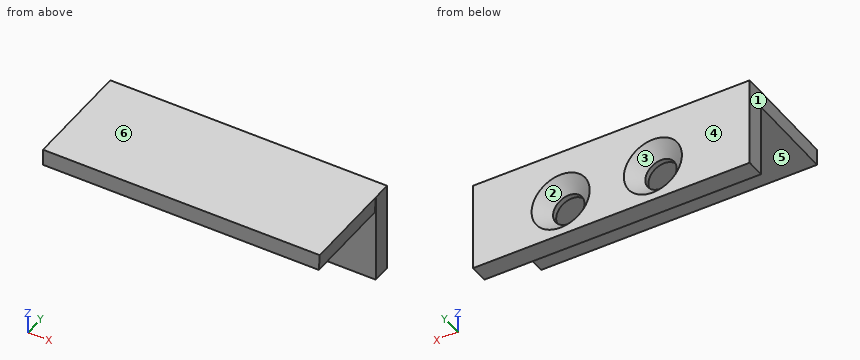
from build123d import *

# Parameters (mm, degrees)
SKIZZE1_W                                            = 30
SKIZZE1_H                                            = 9.8
AUFSATZ_LINEAR_AUSTRAGEN1_DEPTH                      = 2
FORMSENKUNG_F_R_M3_LINSENSENKSCHRAUBE_MI_D           = 3.4
FORMSENKUNG_F_R_M3_LINSENSENKSCHRAUBE_MI_DEPTH       = 8.5
FORMSENKUNG_F_R_M3_LINSENSENKSCHRAUBE_MI_CSINK_D     = 6.3
FORMSENKUNG_F_R_M3_LINSENSENKSCHRAUBE_MI_CSINK_ANGLE = 90
FORMSENKUNG_F_R_M3_LINSENSENKSCHRAUBE_MI_TIP         = 1.021463052
AUFSATZ_LINEAR_AUSTRAGEN2_DEPTH                      = 10


with BuildPart() as part:
    # Skizze1 → Aufsatz-Linear austragen1 (new body)
    with BuildSketch(Plane(origin=(0, 0, 0), x_dir=(1, 0, 0), z_dir=(0, 1, 0))):
        with Locations((5, 8.1)):
            Rectangle(SKIZZE1_W, SKIZZE1_H)
    extrude(amount=AUFSATZ_LINEAR_AUSTRAGEN1_DEPTH)

    # Formsenkung für M3 Linsensenkschraube mit Schlitz1
    with Locations(Plane(origin=(0, 2, 0), x_dir=(1, 0, 0), z_dir=(0, 1, 0))):
        with Locations((0.5, 9), (10.5, 9)):
            CounterSinkHole(FORMSENKUNG_F_R_M3_LINSENSENKSCHRAUBE_MI_D / 2, FORMSENKUNG_F_R_M3_LINSENSENKSCHRAUBE_MI_CSINK_D / 2, depth=FORMSENKUNG_F_R_M3_LINSENSENKSCHRAUBE_MI_DEPTH, counter_sink_angle=FORMSENKUNG_F_R_M3_LINSENSENKSCHRAUBE_MI_CSINK_ANGLE)
            with Locations((0, 0, -(FORMSENKUNG_F_R_M3_LINSENSENKSCHRAUBE_MI_DEPTH + FORMSENKUNG_F_R_M3_LINSENSENKSCHRAUBE_MI_TIP / 2))):  # 118° drill point
                Cone(0, FORMSENKUNG_F_R_M3_LINSENSENKSCHRAUBE_MI_D / 2, FORMSENKUNG_F_R_M3_LINSENSENKSCHRAUBE_MI_TIP, mode=Mode.SUBTRACT)

    # Skizze13 → Aufsatz-Linear austragen2 (add)
    with BuildSketch(Plane.XZ):
        Polygon((-10, -3.2), (-10, -4.99756301), (19.906366545, -4.99756301), (20, -3.2), align=None)
    extrude(amount=AUFSATZ_LINEAR_AUSTRAGEN2_DEPTH)


solid = part.part
For this review, take the finished solid that the model builds, in its own axes (mm). Face numbers are marked on the shaded views. A direction names the side the tool comes from. Give positions to 0.01 mm unless a question says otherwise; leave off trailing zeros. Loops run counter-clockwise (first coordinate to the right, second up) from the corner with the lowest first, then second, coordinate; pieces in that order, holes last. Notation, with made-up numbers: M 69.5,79.5 L 127.5,79.5 A20 cw 127.5,109.5 Z; hole C 76.5,55.25 d7. An arc over 180 degrees is marked long. Put each result on its own line as item: value. Start each with the question number.
(1) Wall thickness on L1, parallel to X at y = 0.25, z = -9; L2, parallel to Z at x = 10.5, y = 0.3; L3, parallel to Y at x = 13.5, z = -10.5: over which ranges is each line inside the solid? List them lowest first.
(2) The part is to be moulded in two halves that separate along X. For the marked faces 1, 2, 3 and 4, say which applies: +X half, -X half, draft (parallel to the pull), parting line (faces both ways), or undercut.
(3) Add section A-A, the plane x = 10.5. Write out the cut boundary in (y, z).
(4) For pin 1 (4 mm diameter, centred on y = -2.5, z = -4.5, fed in from +X); pin 2 (3 mm diameter, centred on x = -2, z = -9, fed in from -Y); pin 3 (5.5 mm diameter, centred on x = 0.5, z = -9, fed in from +Y), all flat-tipped, find the tip position at first contact; note any pin that passes through.
(5) Add section D-D, the plane y = -5.75. Write out the cut boundary in (x, z), then the cut area to 3 significant figures.
(6) Machinability: for the marked faces 5 and 6, which of the approach directions +Z, -Z, +X, -X, +Y, -Y give a long, thin tool a straight path to every point of the face, cutting with its end or side? Answer none if there is none.
(7) Add section C-C, the plane x = -3. Write out the cut boundary in (y, z).
(8) Add section B-B, the plane z = -9. Write out the cut boundary in (x, y), then the cut area to 3 significant figures.
Result:
1. L1: x = -10 to -1.2, 2.2 to 8.8, 12.2 to 20
1. L2: z = -13 to -10.7, -7.3 to -3.2
1. L3: y = 0 to 2
2. face 1: -X half
2. face 2: undercut
2. face 3: undercut
2. face 4: draft
3. outline: M -10,-5 L 0,-5 L 0,-7.3 L 0.55,-7.3 L 2,-5.85 L 2,-3.2 L -10,-3.2 Z; M 0,-13 L 2,-13 L 2,-12.15 L 0.55,-10.7 L 0,-10.7 Z
4. pin 1: stops at x = 20
4. pin 2: stops at y = 0
4. pin 3: stops at y = 1.6
5. outline: M -10,-5 L 19.91,-5 L 20,-3.2 L -10,-3.2 Z
5. area: 53.8 mm^2
6. face 5: -Z, +X, -X, -Y
6. face 6: +Z, +X, -X, +Y, -Y
7. outline: M -10,-5 L 0,-5 L 0,-13 L 2,-13 L 2,-3.2 L -10,-3.2 Z
8. outline: M -10,0 L -1.2,0 L -1.2,0.55 L -2.65,2 L -10,2 Z; M 2.2,0 L 8.8,0 L 8.8,0.55 L 7.35,2 L 3.65,2 L 2.2,0.55 Z; M 12.2,0 L 20,0 L 20,2 L 13.65,2 L 12.2,0.55 Z
8. area: 42.2 mm^2
